The model under review builds one solid part; all positions refer to its coordinate system, in mm. A direction names the side the tool comes from. Give positions to 0.01 mm unless a question says otherwise; leave off trailing zeros. Order: outer loops, then holes, each group sorted by start corner. A loop starts at its lowest first (then second) coordinate and runs counter-clockwise, first axis right, second up. Notation, with made-up numbers: (-3, 48.25) - (14, 48.25) arc R13 cw to (14, 71.25) - close; hole circle Ø5 at (-34, 65.5). An arc over 180 degrees is marked (long way). Put each result on its own line as item: value.
```python
from build123d import *

# Parameters (mm, degrees)
F0_W         = 330.2
F0_H         = 38.1
F1_DEPTH     = 38.1
F2_W         = 19.05
F2_H         = 10.922
F3_DEPTH     = 101.6
F4_W         = 19.05
F4_H         = 10.922
F5_DEPTH     = 101.6
F7_DEPTH     = 22.86
F8_DEPTH     = 10.16
F10_DEPTH    = 7.62
F11_W        = 25.4
F11_H        = 13.589
F11_H_2      = 10.922
F12_DEPTH    = 38.1
F13_T1_DEPTH = 88.9
F13_T3_DEPTH = 88.9
F14_R        = 12.7
F16_DEPTH    = 101.6


# Not quite as in the source:
# - a fillet or chamfer that OpenCascade refuses, or shapes differently, is made with other operations: its cross-section is extruded or revolved along the edge and cut away or added
# - after a boolean that leaves OpenCascade's solid faulty, fix() repairs it
# - a feature names something its author has since deleted; it is built from what else it names


with BuildPart() as f1:
    # F0 (on Top) → F1 (new body)
    with BuildSketch(Plane.XY):
        Rectangle(F0_W, F0_H)
    extrude(amount=F1_DEPTH)

    # F2 (on face) → F3 (cut)
    with BuildSketch(Plane(origin=(-165.1, 0, 0), x_dir=(0, -1, 0), z_dir=(-1, 0, 0))):
        with Locations((9.525, 19.05)):
            Rectangle(F2_W, F2_H)
        with Locations((-9.525, 19.05)):
            Rectangle(F2_W, F2_H)
    extrude(amount=-F3_DEPTH, mode=Mode.SUBTRACT)

    # F4 (on face) → F5 (cut)
    with BuildSketch(Plane.YZ.offset(165.1)):
        with Locations((-9.525, 19.05)):
            Rectangle(F4_W, F4_H)
        with Locations((9.525, 19.05)):
            Rectangle(F4_W, F4_H)
    extrude(amount=-F5_DEPTH, mode=Mode.SUBTRACT)

    # F6 (on face) → F7 (cut)
    with BuildSketch(Plane.XY.offset(38.1)):
        with BuildLine():
            Line((-93.98, 12.827), (-93.98, -12.827))
            ThreePointArc((-93.98, -12.827), (-84.9099413177, -9.0700586823), (-81.153, 0))
            ThreePointArc((-81.153, 0), (-84.9099413177, 9.0700586823), (-93.98, 12.827))
        make_face()
        with BuildLine():
            ThreePointArc((-93.98, 12.827), (-106.807, 0), (-93.98, -12.827))
            Line((-93.98, -12.827), (-93.98, 12.827))
        make_face()
        with BuildLine():
            ThreePointArc((93.98, 12.827), (81.153, 0), (93.98, -12.827))
            Line((93.98, -12.827), (93.98, 12.827))
        make_face()
        with BuildLine():
            Line((93.98, 12.827), (93.98, -12.827))
            ThreePointArc((93.98, -12.827), (103.0500586823, -9.0700586823), (106.807, 0))
            ThreePointArc((106.807, 0), (103.0500586823, 9.0700586823), (93.98, 12.827))
        make_face()
    extrude(amount=-F7_DEPTH, mode=Mode.SUBTRACT)

    # F6 (on face) → F8 (join)
    with BuildSketch(Plane.XY.offset(38.1)):
        with BuildLine():
            ThreePointArc((110.7805208253, 19.05), (93.98, 25.4), (77.1794791747, 19.05))
            Line((77.1794791747, 19.05), (93.98, 19.05))
            Line((93.98, 19.05), (110.7805208253, 19.05))
        make_face()
        with BuildLine():
            Line((110.7805208253, -19.05), (147.8615367264, -19.05))
            ThreePointArc((147.8615367264, -19.05), (150.3069576842, -9.6641780842), (151.13, 0))
            ThreePointArc((151.13, 0), (150.3069576842, 9.6641780842), (147.8615367264, 19.05))
            Line((147.8615367264, 19.05), (110.7805208253, 19.05))
            ThreePointArc((110.7805208253, 19.05), (117.1305208253, 10.4505208253), (119.38, 0))
            ThreePointArc((119.38, 0), (117.1305208253, -10.4505208253), (110.7805208253, -19.05))
        make_face()
        with BuildLine():
            ThreePointArc((147.8615367264, 19.05), (93.98, 57.15), (40.0984632736, 19.05))
            Line((40.0984632736, 19.05), (77.1794791747, 19.05))
            ThreePointArc((77.1794791747, 19.05), (93.98, 25.4), (110.7805208253, 19.05))
            Line((110.7805208253, 19.05), (147.8615367264, 19.05))
        make_face()
        with BuildLine():
            ThreePointArc((77.1794791747, 19.05), (68.58, 0), (77.1794791747, -19.05))
            Line((77.1794791747, -19.05), (93.98, -19.05))
            Line((93.98, -19.05), (93.98, -12.827))
            ThreePointArc((93.98, -12.827), (81.153, 0), (93.98, 12.827))
            Line((93.98, 12.827), (93.98, 19.05))
            Line((93.98, 19.05), (77.1794791747, 19.05))
        make_face()
        with BuildLine():
            Line((93.98, -19.05), (110.7805208253, -19.05))
            ThreePointArc((110.7805208253, -19.05), (117.1305208253, -10.4505208253), (119.38, 0))
            ThreePointArc((119.38, 0), (117.1305208253, 10.4505208253), (110.7805208253, 19.05))
            Line((110.7805208253, 19.05), (93.98, 19.05))
            Line((93.98, 19.05), (93.98, 12.827))
            ThreePointArc((93.98, 12.827), (103.0500586823, 9.0700586823), (106.807, 0))
            ThreePointArc((106.807, 0), (103.0500586823, -9.0700586823), (93.98, -12.827))
            Line((93.98, -12.827), (93.98, -19.05))
        make_face()
        with BuildLine():
            ThreePointArc((40.0984632736, 19.05), (36.83, 0), (40.0984632736, -19.05))
            Line((40.0984632736, -19.05), (77.1794791747, -19.05))
            ThreePointArc((77.1794791747, -19.05), (68.58, 0), (77.1794791747, 19.05))
            Line((77.1794791747, 19.05), (40.0984632736, 19.05))
        make_face()
        with BuildLine():
            Line((77.1794791747, -19.05), (40.0984632736, -19.05))
            ThreePointArc((40.0984632736, -19.05), (93.98, -57.15), (147.8615367264, -19.05))
            Line((147.8615367264, -19.05), (110.7805208253, -19.05))
            ThreePointArc((110.7805208253, -19.05), (93.98, -25.4), (77.1794791747, -19.05))
        make_face()
        with BuildLine():
            Line((93.98, -19.05), (77.1794791747, -19.05))
            ThreePointArc((77.1794791747, -19.05), (93.98, -25.4), (110.7805208253, -19.05))
            Line((110.7805208253, -19.05), (93.98, -19.05))
        make_face()
        with BuildLine():
            Line((-93.98, -12.827), (-93.98, -19.05))
            Line((-93.98, -19.05), (-40.0984632736, -19.05))
            ThreePointArc((-40.0984632736, -19.05), (-37.6530423158, -9.6641780842), (-36.83, 0))
            ThreePointArc((-36.83, 0), (-37.6530423158, 9.6641780842), (-40.0984632736, 19.05))
            Line((-40.0984632736, 19.05), (-93.98, 19.05))
            Line((-93.98, 19.05), (-93.98, 12.827))
            ThreePointArc((-93.98, 12.827), (-84.9099413177, 9.0700586823), (-81.153, 0))
            ThreePointArc((-81.153, 0), (-84.9099413177, -9.0700586823), (-93.98, -12.827))
        make_face()
        with BuildLine():
            Line((-147.8615367264, -19.05), (-93.98, -19.05))
            Line((-93.98, -19.05), (-93.98, -12.827))
            ThreePointArc((-93.98, -12.827), (-106.807, 0), (-93.98, 12.827))
            Line((-93.98, 12.827), (-93.98, 19.05))
            Line((-93.98, 19.05), (-147.8615367264, 19.05))
            ThreePointArc((-147.8615367264, 19.05), (-151.13, 0), (-147.8615367264, -19.05))
        make_face()
        with BuildLine():
            Line((-40.0984632736, -19.05), (-93.98, -19.05))
            Line((-93.98, -19.05), (-147.8615367264, -19.05))
            ThreePointArc((-147.8615367264, -19.05), (-93.98, -57.15), (-40.0984632736, -19.05))
        make_face()
        with BuildLine():
            ThreePointArc((-40.0984632736, 19.05), (-93.98, 57.15), (-147.8615367264, 19.05))
            Line((-147.8615367264, 19.05), (-93.98, 19.05))
            Line((-93.98, 19.05), (-40.0984632736, 19.05))
        make_face()
    extrude(amount=F8_DEPTH)

    # F9 (on face) → F10 (join)
    with BuildSketch(Plane.XZ.offset(19.05)):
        Polygon((0, 0), (0, 38.1), (-40.0984632736, 38.1), (-63.5, 38.1), (-63.5, 30.861), (-63.5, 24.511), (-63.5, 19.939), (-63.5, 13.589), (-63.5, 0), align=None)
        Polygon((63.5, 30.861), (63.5, 38.1), (40.0984632736, 38.1), (13.5538854515, 38.1), (0, 38.1), (0, 0), (63.5, 0), (63.5, 13.589), (63.5, 19.939), (63.5, 24.511), align=None)
    extrude(amount=F10_DEPTH)

    add(f1.part.fix(), mode=Mode.REPLACE)

    # F11 (on face) → F12 (join)
    with BuildSketch(Plane(origin=(0, 19.05, 0), x_dir=(-1, 0, 0), z_dir=(0, 1, 0))):
        with Locations((-27.3984632736, 31.3055)):
            Rectangle(F11_W, F11_H)
        with Locations((-27.3984632736, 19.05)):
            Rectangle(F11_W, F11_H_2)
        with Locations((27.3984632736, 19.05)):
            Rectangle(F11_W, F11_H_2)
        with Locations((27.3984632736, 31.3055)):
            Rectangle(F11_W, F11_H)
    extrude(amount=F12_DEPTH)

    # F13: fillet of radius 12.7 on 2 edges, made by hand

    # F13_s2 → F13_t1 (cut)
    with BuildSketch(Plane.YZ.offset(-71.8484632736)):
        with BuildLine():
            add(Edge.make_bspline(
                [(44.45, 13.589), (57.15, 13.589), (57.15, 26.289)],
                knots=[0, 0, 0, 1, 1, 1], degree=2, weights=[1, 1, 1]))
            Line((57.15, 26.289), (57.15, 13.589))
            Line((57.15, 13.589), (44.45, 13.589))
        make_face()
    extrude(amount=F13_T1_DEPTH, mode=Mode.SUBTRACT)

    # F13_s4 → F13_t3 (cut)
    with BuildSketch(Plane.YZ.offset(-17.0515367264)):
        with BuildLine():
            add(Edge.make_bspline(
                [(44.45, 13.589), (57.15, 13.589), (57.15, 26.289)],
                knots=[0, 0, 0, 1, 1, 1], degree=2, weights=[1, 1, 1]))
            Line((57.15, 26.289), (57.15, 13.589))
            Line((57.15, 13.589), (44.45, 13.589))
        make_face()
    extrude(amount=F13_T3_DEPTH, mode=Mode.SUBTRACT)

    # F14
    f14_edges = [f1.edges().sort_by_distance(p)[0] for p in [
        (27.398463, 57.15, 38.1),
        (-27.398463, 57.15, 38.1),
    ]]
    fillet(f14_edges, radius=F14_R)

    # F15 (on face) → F16 (cut)
    with BuildSketch(Plane(origin=(-40.0984632736, 0, 0), x_dir=(0, -1, 0), z_dir=(-1, 0, 0))):
        with BuildLine():
            ThreePointArc((-52.3875, 25.8445), (-44.45, 17.907), (-36.5125, 25.8445))
            Line((-36.5125, 25.8445), (-52.3875, 25.8445))
        make_face()
        with BuildLine():
            Line((-52.3875, 25.8445), (-36.5125, 25.8445))
            ThreePointArc((-36.5125, 25.8445), (-44.45, 33.782), (-52.3875, 25.8445))
        make_face()
    extrude(amount=-F16_DEPTH, mode=Mode.SUBTRACT)


solid = f1.part
```
(1) Take a section at C-C, the plane x = -76.5. Write out the cut boundary in (y, z).
The answers:
outline: (-54.41, 38.1) - (-19.05, 38.1) - (-19.05, 24.51) - (19.05, 24.51) - (19.05, 38.1) - (54.41, 38.1) - (54.41, 48.26) - (-54.41, 48.26) - close; (-19.05, 0) - (19.05, 0) - (19.05, 13.59) - (-19.05, 13.59) - close
(2) Take a section at A-A, the plane z = 45. Write out the cut boundary in (x, y), then the cut area to 3 significant figures.
The answers:
outline: circle Ø114.3 at (-93.98, 0); circle Ø114.3 at (93.98, 0); hole circle Ø25.65 at (-93.98, 0); hole circle Ø25.65 at (93.98, 0)
area: 19,500 mm^2
(3) Wall thickness on L1, parallel to Z at x = 136.5, y = 9; L2, parallel to X at y = -3, z = 25.5; L3, parallel to Z at x = -23, y = 44: over which ranges is each line inside the solid? List them lowest first.
The answers:
L1: 0 to 13.59, 24.51 to 48.26
L2: -165.1 to -106.45, -81.51 to 81.51, 106.45 to 165.1
L3: 13.59 to 17.92, 33.77 to 38.1
(4) The part is to be moulded in two halves that separate along Y. For faces 1 (the flat face through (-2, 19.05, 19)), 2 (the flat face through (-95, 14, 48.26)), 3 (the cylindrical face through (-27.576, 50.749, 21.015)), say which applies: pulls with the +Y half, pulls with the -Y half, needs draft (parallel to the pull), parting line crosses it, or undercut.
The answers:
face 1: pulls with the +Y half
face 2: needs draft
face 3: undercut
(5) Take a section at B-B, the plane y = -37.5. Write out the cut boundary in (x, z).
The answers:
outline: (-137.11, 38.1) - (-50.85, 38.1) - (-50.85, 48.26) - (-137.11, 48.26) - close; (50.85, 38.1) - (137.11, 38.1) - (137.11, 48.26) - (50.85, 48.26) - close
(6) For faces 4 (the flat face through (28, 32, 13.589)), 5 (the flat face through (-95, 34, 38.1)), 6 (the flat face through (-115, 0, 13.589)), list the 3-axis set-ups (+Z, -Z, +X, -X, +Y, -Y) from which the entire face can be reached by the end or side of a thin tool; tool diameter is ignored.
The answers:
face 4: -Z, +X, -X, +Y
face 5: -Z, -X, +Y
face 6: -X, +Y, -Y
(7) Clearance check with flat-ended pins moving along their axes: pin 1 Ø4 at (x, z) = (136, 32.5) entering from -Y; pin 2 Ø1.5 at (y, z) = (33, 18) entering from -X; pin 3 Ø10 at (x, z) = (-31.5, 21.5) entering from -Y; pin 4 Ø14.5 at (y, z) = (44.45, 25.84) entering from +X. State where each tip first meets the part, or that it passes through.
The answers:
pin 1: y = -19.05
pin 2: x = -40.1
pin 3: y = -26.67
pin 4: through
(8) Take a section at D-D, the plane y = 40. Write out the cut boundary in (x, z), then the cut area to 3 significant figures.
The answers:
outline: (-134.8, 38.1) - (-53.16, 38.1) - (-53.16, 48.26) - (-134.8, 48.26) - close; (-40.1, 13.59) - (-14.7, 13.59) - (-14.7, 19.27) - (-40.1, 19.27) - close; (-40.1, 32.42) - (-14.7, 32.42) - (-14.7, 38.1) - (-40.1, 38.1) - close; (14.7, 13.59) - (40.1, 13.59) - (40.1, 19.27) - (14.7, 19.27) - close; (14.7, 32.42) - (40.1, 32.42) - (40.1, 38.1) - (14.7, 38.1) - close; (53.16, 38.1) - (134.8, 38.1) - (134.8, 48.26) - (53.16, 48.26) - close
area: 2,240 mm^2
